For this review, take the finished solid that the model builds, in its own axes (mm). Face numbers are marked on the shaded views. A direction names the side the tool comes from. Coordinates: 2 decimals unless noted, no trailing zeros. Loops run counter-clockwise (first coordinate to the right, second up) from the corner with the lowest first, then second, coordinate; pieces in that order, holes last. Notation, with made-up numbers: (61.25, 60.25) -> (80.25, 60.25) arc R26 cw to (80.25, 74.25) -> close; hole circle Ø3 at (28, 8). An arc over 180 degrees is marked (long way). Use a Markdown table: item, result.
Solid Edge part; units mm, degrees
sketch "Sketch1" plane through (0, 0, 0) normal (0, 0, 1) x (1, 0, 0)
  line L0 (-46.5, -60) -> (46.5, -60)
  line L1 (46.5, -60) -> (46.5, 60)
  line L2 (46.5, 60) -> (-46.5, 60)
  line L3 (-46.5, 60) -> (-46.5, -60)
extrude "Protrusion1" add sketch "Sketch1" along normal blind 2
sketch "Sketch2" plane through (0, 0, 2) normal (0, 0, 1) x (1, 0, 0)
  line L0 (-35.5, -15.5) -> (35.5, -15.5)
  line L1 (35.5, -15.5) -> (35.5, 15.5)
  line L2 (35.5, 15.5) -> (-35.5, 15.5)
  line L3 (-35.5, 15.5) -> (-35.5, -15.5)
extrude "Cutout1" cut sketch "Sketch2" against normal up to next
sketch "Sketch3" plane through (0, 0, 2) normal (0, 0, 1) x (1, 0, 0)
  line L0 (-35.5, 22.293) -> (35.5, 22.293)
  line L1 (35.5, 22.293) -> (35.5, 27.293)
  line L2 (35.5, 27.293) -> (-35.5, 27.293)
  line L3 (-35.5, 27.293) -> (-35.5, 22.293)
extrude "Cutout2" cut sketch "Sketch3" against normal up to next
sketch "Sketch4" plane through (0, 0, 2) normal (0, 0, 1) x (1, 0, 0)
  line L0 (11.5, -25.6896) -> (-11.5, -25.6896)
  line L1 (-11.5, -25.6896) -> (-11.5, -48.6896)
  line L2 (-11.5, -48.6896) -> (11.5, -48.6896)
  line L3 (11.5, -48.6896) -> (11.5, -25.6896)
extrude "Cutout3" cut sketch "Sketch4" against normal up to next
sketch "Sketch5" plane through (0, 0, 2) normal (0, 0, 1) x (1, 0, 0)
  line L0 (-12.5, -24.6896) -> (-12.5, -49.6896)
  line L1 (-12.5, -49.6896) -> (12.5, -49.6896)
  line L2 (12.5, -49.6896) -> (12.5, -24.6896)
  line L3 (12.5, -24.6896) -> (-12.5, -24.6896)
  line L4 (-11.5, -25.6896) -> (-11.5, -48.6896)
  line L5 (-11.5, -48.6896) -> (11.5, -48.6896)
  line L6 (11.5, -48.6896) -> (11.5, -25.6896)
  line L7 (11.5, -25.6896) -> (-11.5, -25.6896)
extrude "Protrusion2" add sketch "Sketch5" against normal blind 20
sketch "Sketch6" plane through (0, 0, 2) normal (0, 0, 1) x (1, 0, 0)
  arc A0 (-34.5, -37.1896) -> (-24.5, -37.1896) centre (-29.5, -37.1896) cw
  line L0 (-34.5, -37.1896) -> (-34.5, -58)
  line L1 (-24.5, -58) -> (-24.5, -37.1896)
  line L2 (-34.5, -58) -> (-24.5, -58)
extrude "Cutout4" cut sketch "Sketch6" against normal up to next
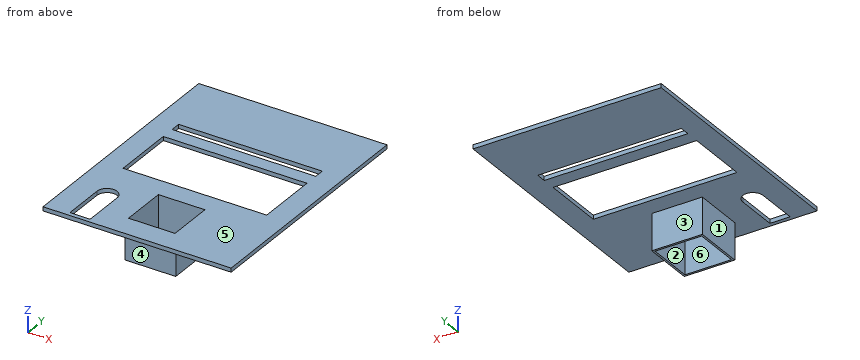
(1) Take a section at B-B on x = -23. Write out the cut boundary in (y, z).
Found:
| item | result |
|---|---|
| outline | (-60, 0) -> (-15.5, 0) -> (-15.5, 2) -> (-60, 2) -> close; (15.5, 0) -> (22.29, 0) -> (22.29, 2) -> (15.5, 2) -> close; (27.29, 0) -> (60, 0) -> (60, 2) -> (27.29, 2) -> close |
(2) For the marked faces 4, 5 and 6, list the 3-axis set-ups (+Z, -Z, +X, -X, +Y, -Y) from which the entire face can be reached by the end or side of a thin tool; tool diameter is ignored.
Found:
| item | result |
|---|---|
| face 4 | -Z, +X, -X, -Y |
| face 5 | +Z, +X, -X, +Y, -Y |
| face 6 | +Z, -Z |
(3) For line 1 along Y through (x, z) = (0.5, 0.75); line 2 along Y through (x, z) = (34, 1.25); line 3 along Y through (x, z) = (5, -4.5), list the stretches that pass through material, from the lowest coordinate up.
Found:
| item | result |
|---|---|
| line 1 | y = -60 to -48.69, -25.69 to -15.5, 15.5 to 22.29, 27.29 to 60 |
| line 2 | y = -60 to -15.5, 15.5 to 22.29, 27.29 to 60 |
| line 3 | y = -49.69 to -48.69, -25.69 to -24.69 |
(4) Mouldability with a two-part tool opening along X and no side actions: class the marked faces 1, 2 and 3 as pulls with the +X half, pulls with the -X half, needs draft (parallel to the pull), parting line crosses it, or undercut.
Found:
| item | result |
|---|---|
| face 1 | pulls with the -X half |
| face 2 | undercut |
| face 3 | needs draft |
(5) Take a section at C-C on y = -27. Write out the cut boundary in (x, z), plus the area to 3 significant figures.
Found:
| item | result |
|---|---|
| outline | (-46.5, 0) -> (-12.5, 0) -> (-12.5, -18) -> (-11.5, -18) -> (-11.5, 2) -> (-46.5, 2) -> close; (11.5, -18) -> (12.5, -18) -> (12.5, 0) -> (46.5, 0) -> (46.5, 2) -> (11.5, 2) -> close |
| area | 176 mm^2 |
(6) For pin 1 Ø8 at (y, z) = (-22, -13.5) entering from -X; pin 2 Ø10 at (x, z) = (15.5, -1) entering from +Y; pin 3 Ø1.5 at (x, y) = (21, -32) entering from -Z; pin 4 Ø9 at (x, z) = (0, -12) entering from -Y, all flat-tipped, find the tip position at first contact; note any pin that passes through.
Found:
| item | result |
|---|---|
| pin 1 | stops at x = -12.5 |
| pin 2 | stops at y = 60 |
| pin 3 | stops at z = 0 |
| pin 4 | stops at y = -49.69 |
(7) Take a section at A-A on x = -1. Write out the cut boundary in (y, z).
Found:
| item | result |
|---|---|
| outline | (-60, 0) -> (-49.69, 0) -> (-49.69, -18) -> (-48.69, -18) -> (-48.69, 2) -> (-60, 2) -> close; (-25.69, -18) -> (-24.69, -18) -> (-24.69, 0) -> (-15.5, 0) -> (-15.5, 2) -> (-25.69, 2) -> close; (15.5, 0) -> (22.29, 0) -> (22.29, 2) -> (15.5, 2) -> close; (27.29, 0) -> (60, 0) -> (60, 2) -> (27.29, 2) -> close |
(8) Take a section at D-D on z = -14.5. Write out the cut boundary in (x, y).
Found:
| item | result |
|---|---|
| outline | (-12.5, -49.69) -> (12.5, -49.69) -> (12.5, -24.69) -> (-12.5, -24.69) -> close; hole (-11.5, -48.69) -> (11.5, -48.69) -> (11.5, -25.69) -> (-11.5, -25.69) -> close |
